Autodesk Fusion 360 part; units mm, degrees
sketch "Sketch1" plane through (0, 0, 0) normal (1, 0, 0) x (0, 1, 0)
  line L0 (0, 0) -> (0, 51)
  line L1 (0, 0) -> (127, 0)
  line L2 (127, 0) -> (127, 0.0001)
  line L3 (0, 51) -> (2.5, 51)
  line L4 (37.5, 7.5) -> (119.5, 7.5)
  line L5 (-5, 0) -> (-5, 33)
  line L6 (69.5, -10) -> (108, -10)
  line L7 (15, 30) -> (15, 38.5)
  arc A0 (15, 38.5) -> (2.5, 51) centre (2.5, 38.5) ccw
  arc A1 (127, 0.0001) -> (119.5, 7.5) centre (119.5, 0) ccw
  arc A2 (15, 30) -> (37.5, 7.5) centre (37.5, 30) ccw
  point P0 (126.9999, 7.5)
  point P1 (15, 51)
  point P2 (15, 7.5)
  dimension "d1" = 51
  dimension "d2" = 127
  dimension "d5" = 7.5
  dimension "d6" = 43.5
  dimension "d7" = 33
  dimension "d10" = 12.5
  dimension "d11" = 7.5
  dimension "d12" = 22.5
sketch "Sketch2" plane through (0, 0, 0) normal (0, 0, 1) x (1, 0, 0)
  circle A0 centre (0, 69.5) radius 3.375
  circle A1 centre (0, 108) radius 3.875
  dimension "d13" = 6.75
  dimension "d14" = 7.75
sketch "Sketch3" plane through (0, 0, 0) normal (0, 1, 0) x (1, 0, 0)
  circle A0 centre (0, -30) radius 5.1
  circle A1 centre (0, -30) radius 11.15
  dimension "d15" = 10.2
  dimension "d16" = 22.3
extrude "Extrude1" add sketch "Sketch1" along normal mid plane 26
extrude "Extrude2" cut sketch "Sketch2" along normal blind 20
extrude "Extrude3" cut sketch "Sketch3" along normal blind 90 contours A0
extrude "Extrude4" cut sketch "Sketch3" along normal blind 20 from surface at 8.2
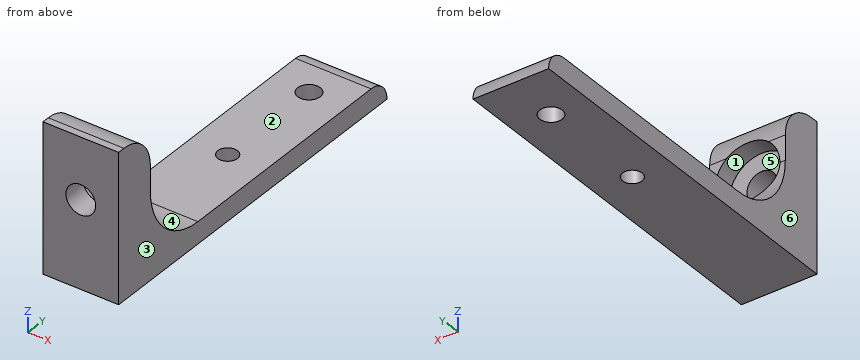
Model file for the job. Use its own axes, mm. Face numbers are marked on the shaded views. A direction names the side the tool comes from. Give positions to 0.01 mm unless a question says otherwise; leave off trailing zeros. Loops run counter-clockwise (first coordinate to the right, second up) from the corner with the lowest first, then second, coordinate; pieces in that order, holes last. Notation, with made-up numbers: M 20,55 L 32,55 A32 ccw 32,93 Z; hole C 65,52.25 d10. An arc over 180 degrees is marked long. Use one line per item in the form item = value.
Item 1: Slice it at A-A on y = 69.5. List the corners of the cut face in (x, z) (3 decimals).
Filled in:
outline = M -13,0 L -3.375,0 L -3.375,7.5 L -13,7.5 Z; M 3.375,0 L 13,0 L 13,7.5 L 3.375,7.5 Z
Item 2: Two-plate mould, pull along Z, no slides. Class the marked faces 4, 5 and 6: released by +Z, released by -Z, zero draft, split by the parting line, or undercut.
Filled in:
face_4 = released by +Z
face_5 = undercut
face_6 = zero draft
Item 3: Slice it at B-B on z = 4.5. List the corners of the cut face in (x, y) (3 decimals), and give its area (3 significant figures).
Filled in:
outline = M -13,0 L 13,0 L 13,125.5 L -13,125.5 Z; hole C 0,108 d7.75; hole C 0,69.5 d6.75
area = 3,180 mm^2
Item 4: Which spindle directions (+Z, -Z, +X, -X, +Y, -Y) get a long thin tool onto all of the face, cutting with end or side? Do the marked faces 1, 2 and 3. Say none if no direction does.
Filled in:
face_1 = +Y
face_2 = +Z, +X, -X, +Y
face_3 = +Z, -Z, +X, +Y, -Y
Item 5: Slice it at D-D on z = 37. List the corners of the cut face in (x, y), and give its area (3 significant figures).
Filled in:
outline = M -13,0 L 13,0 L 13,15 L 8.68,15 L 8.68,8.2 L -8.68,8.2 L -8.68,15 L -13,15 Z
area = 272 mm^2
Item 6: Flat gauge pins, fed straight in: pin 1 Ø1 at (x, y) = (-8, 57) entering from +Z; pin 2 Ø9 at (x, y) = (0, 69.5) entering from -Z; pin 3 Ø3 at (x, z) = (11.5, 33) entering from +Y; pin 4 Ø13.5 at (x, z) = (0, 30) entering from +Y. Where does each tip first touch, or does it go through?
Filled in:
pin_1 = 7.5
pin_2 = 0
pin_3 = 15
pin_4 = 8.2
Item 7: Slice it at C-C on x = 1. List the corners of the cut face in (y, z).
Filled in:
outline = M 0,0 L 66.28,0 L 66.28,7.5 L 37.5,7.5 A22.5 cw 17.93,18.89 L 8.2,18.89 L 8.2,25 L 0,25 Z; M 0,35 L 8.2,35 L 8.2,41.11 L 14.73,41.11 A12.5 ccw 2.5,51 L 0,51 Z; M 72.72,0 L 104.26,0 L 104.26,7.5 L 72.72,7.5 Z; M 111.74,0 L 127,0 A7.5 ccw 119.5,7.5 L 111.74,7.5 Z
Item 8: Drill centre lines: L1, parallel to Y at x = 0, z = 5.5 (3 decimals); L2, parallel to X at y = 108, z = 2.25 (3 decimals); L3, parallel to X at y = 14.25, z = 30. Where is each one in solid material? Low to high.
Filled in:
L1 = 0 to 66.125, 72.875 to 104.125, 111.875 to 124.599
L2 = -13 to -3.875, 3.875 to 13
L3 = -13 to -11.15, 11.15 to 13
